Autodesk Inventor part; units mm, degrees
ref_plane "YZ Plane" through (0, 0, 0) normal (1, 0, 0) x (0, 1, 0)
ref_plane "XZ Plane" through (0, 0, 0) normal (0, 1, 0) x (-1, 0, 0)
ref_plane "XY Plane" through (0, 0, 0) normal (0, 0, 1) x (1, 0, 0)
sketch "Boceto6" plane through (0, 0, 0) normal (0, 1, 0) x (-1, 0, 0)
  line L0 (-51.5, -51.5) -> (51.5, -51.5)
  line L1 (51.5, -51.5) -> (51.5, 51.5)
  line L2 (51.5, 51.5) -> (-51.5, 51.5)
  line L3 (-51.5, 51.5) -> (-51.5, -51.5)
  line L4 (-53.9142, 52.5) -> (52.5, 52.5)
  line L5 (52.5, 52.5) -> (52.5, -53.9142)
  line L6 (52.5, 53.9142) -> (52.5, -52.5)
  line L7 (52.5, -52.5) -> (-53.9142, -52.5)
  arc A0 (-21.9085, 20.4943) -> (-21.9085, -20.4943) centre (0, 0) ccw
  line L8 (-53.9142, -52.5) -> (-51.5, -50.0858)
  line L9 (-21.9085, -20.4943) -> (-7.0317, -5.6174)
  line L10 (-7.0317, 5.6174) -> (-21.9085, 20.4943)
  line L11 (-51.5, 50.0858) -> (-53.9142, 52.5)
  circle A1 centre (0, 0) radius 4.1
  arc A2 (-7.0317, 5.6174) -> (-7.0317, -5.6174) centre (0, 0) ccw
  dimension "d32" = 103
  dimension "d33" = 103
  dimension "d39" = 8.2
  dimension "d49" = 18
extrude "Extrusión4" add sketch "Boceto6" along normal blind 3 contours L3 L2 L1 L0
sketch "Boceto7" plane through (0, 3, 0) normal (0, 1, 0) x (1, 0, 0)
  circle A0 centre (39.5, 0) radius 1.5
  circle A1 centre (0, 39.5) radius 1.5
  line L0 (51.5, -51.5) -> (51.5, 51.5)
  line L1 (-51.5, -51.5) -> (51.5, -51.5)
  line L2 (-51.5, 51.5) -> (-51.5, -51.5)
  line L3 (51.5, 51.5) -> (-51.5, 51.5)
  arc A2 (-5.9631, 4.5488) -> (-5.9631, -4.5488) centre (0, 0) ccw
  line L4 (-21.9085, 20.4943) -> (-5.9631, 4.5488)
  arc A3 (-21.9085, 20.4943) -> (-21.9085, -20.4943) centre (0, 0) ccw
  line L5 (-5.9631, -4.5488) -> (-21.9085, -20.4943)
  circle A4 centre (-39.5, 0) radius 1.5
  circle A5 centre (0, -39.5) radius 1.5
  point P0 (0, 0)
hole "Agujero3" at (39.5, 3, 0) at (0, 3, -39.5) at (-39.5, 3, 0) at (0, 3, 39.5) direction (0, -1, 0) diameter 3 end through all
sketch "Boceto8" plane through (0, 3, 0) normal (0, 1, 0) x (1, 0, 0)
  line L0 (51.5, -51.5) -> (51.5, -21.5)
  line L1 (51.5, -51.5) -> (51.5, 51.5)
  line L2 (51.5, -21.5) -> (39.7367, -21.5)
  line L3 (39.7367, -21.5) -> (39.7367, 25.2431)
  line L4 (39.7367, 25.2431) -> (51.5, 25.2431)
  line L5 (51.5, 25.2431) -> (51.5, -21.5)
  point P0 (0, 0)
  dimension "d50" = 30
extrude "Extrusión5" cut sketch "Boceto8" against normal blind 10
properties part number "Plataforma"
The listing builds one solid part. Answer for the finished solid, in the listing's coordinates (mm). A direction names the side the tool comes from. Coordinates: 2 decimals unless noted, no trailing zeros. Write each loop counter-clockwise with the first axis right and the second up, starting at its lowest first coordinate (ties: lowest second). Pieces come first, ordered by that corner, then holes. Notation, with made-up numbers: (-29, 65) - (-2, 65) arc R9 ccw to (-2, 76) - close; hole circle Ø3 at (-2, -36). An arc over 180 degrees is marked (long way). Return JSON: item names as keys, results as strings. Group by question number.
1. A cutting plane is placed at C-C, the plane y = 2. Determine the outline of the cut face in (x, z), plus the area to 3 significant figures.
2. A cutting plane is placed at A-A, the plane x = 0. Determine the outline of the cut face in (y, z), plus the area to 3 significant figures.
3. Straight lines are drawn through the part: L1, parallel to X at y = 1.1, z = 39.5; L2, parallel to Z at x = 0, y = 1.7; L3, parallel to Z at x = 44.5, y = 1.85. For each, find the intervals that lie inside material, in ascending order.
4. A cutting plane is placed at B-B, the plane z = 0. Determine the outline of the cut face in (x, y), plus the area to 3 significant figures.
5. Determine the mould class of faces 4 (the flat face through (-1, 1, 51.5)), 5 (the flat face through (46, 2, -25.243)), 6 (the flat face through (51.5, 1, -38)), 7 (the flat face through (46, 2, 21.5)) for opening direction Z: released by +Z, released by -Z, zero draft, split by the parting line, or undercut.
6. Given pin 1 (4 mm diameter, centred on x = 0, z = 39.5, fed in from +Y); pin 2 (1.5 mm diameter, centred on y = 1, z = 9, fed in from +X), each flat-ended and moving along its own axis, determine where each tip first touches the part or whether it passes through.
7. Which of the six approach directions +Z, -Z, +X, -X, +Y, -Y give full straight-line access (tool end or side, diameter ignored) to faces 1 (the flat face through (-51.5, 1, -1)), 2 (the cylindrical face through (9, 1, 0)), 3 (the flat face through (39.737, 2, -13))?
8. A cutting plane is placed at D-D, the plane x = 44. Determine the outline of the cut face in (y, z), plus the area to 3 significant figures.
Ans:
{
 "1": {"outline": "(-51.5, -51.5) - (51.5, -51.5) - (51.5, -25.24) - (39.74, -25.24) - (39.74, -1.48) arc R1.5 cw (long way) to (39.74, 1.48) - (39.74, 21.5) - (51.5, 21.5) - (51.5, 51.5) - (-51.5, 51.5) - close; hole circle Ø3 at (-39.5, 0); hole circle Ø8.2 at (0, 0); hole circle Ø3 at (0, -39.5); hole circle Ø3 at (0, 39.5); hole (7.03, -5.62) - (21.91, -20.49) arc R30 ccw to (21.91, 20.49) - (7.03, 5.62) arc R9 cw to start", "area": "9,380 mm²"},
 "2": {"outline": "(0, -51.5) - (3, -51.5) - (3, -41) - (0, -41) - close; (0, -38) - (3, -38) - (3, -4.1) - (0, -4.1) - close; (0, 4.1) - (3, 4.1) - (3, 38) - (0, 38) - close; (0, 41) - (3, 41) - (3, 51.5) - (0, 51.5) - close", "area": "266 mm²"},
 "3": {"L1": "-51.5 to -1.5, 1.5 to 51.5", "L2": "-51.5 to -41, -38 to -4.1, 4.1 to 38, 41 to 51.5", "L3": "-51.5 to -25.24, 21.5 to 51.5"},
 "4": {"outline": "(-51.5, 0) - (-41, 0) - (-41, 3) - (-51.5, 3) - close; (-38, 0) - (-4.1, 0) - (-4.1, 3) - (-38, 3) - close; (4.1, 0) - (9, 0) - (9, 3) - (4.1, 3) - close; (30, 0) - (38, 0) - (38, 3) - (30, 3) - close", "area": "172 mm²"},
 "5": {"face 4": "released by +Z", "face 5": "undercut", "face 6": "zero draft", "face 7": "undercut"},
 "6": {"pin 1": "y = 3", "pin 2": "x = 39.74"},
 "7": {"face 1": "+Z, -Z, -X, +Y, -Y", "face 2": "+Y, -Y", "face 3": "+X, +Y, -Y"},
 "8": {"outline": "(0, -51.5) - (3, -51.5) - (3, -25.24) - (0, -25.24) - close; (0, 21.5) - (3, 21.5) - (3, 51.5) - (0, 51.5) - close", "area": "169 mm²"}
}
